CAD build for the part. Positions are in the model's coordinates, mm. Give positions to 0.01 mm unless a question says otherwise; leave off trailing zeros. Write each loop counter-clockwise with the first axis right and the second up, starting at its lowest first coordinate (ties: lowest second). Pieces come first, ordered by that corner, then holes. Notation, with made-up numbers: M -0.75,42 L 32.25,42 A26 cw 32.25,57 Z; hole C -15.75,14.5 d7. An arc over 180 degrees is marked long. One line per question, with ' | ' between items. Start each with the question number.
1. Wall check: L1, parallel to X at y = 0, z = -1.15; L2, parallel to Z at x = 19, y = 150. Give the ranges that are in metal, low to high.
2. Cut at A-A, the plane y = 53. Write the cut outline in (x, z) (3 decimals), then the cut area to 3 significant figures.
3. Flat gauge pins, fed straight in: pin 1 (1.2 mm diameter, centred on x = 18.5, y = 52.5, fed in from +Z); pin 2 (0.9 mm diameter, centred on x = 0, y = 0, fed in from +Z); pin 3 (3 mm diameter, centred on x = 0, y = 177.44, fed in from +Z). Where does each tip first touch, or does it go through?
```python
from build123d import *

# Parameters (mm, degrees)
F0_W     = 49.8404
F0_H     = 183.4444
F0_R     = 1.5
F0_R_2   = 1.375
F1_DEPTH = 0.5
F2_W     = 49.8404
F2_H     = 183.4444
F2_R     = 1.375
F3_DEPTH = 3
F4_W     = 2.381
F4_H     = 183.4444
F5_DEPTH = 0.4


with BuildPart() as f1:
    # F0 (on Top) → F1 (new body)
    with BuildSketch(Plane.XY):
        with Locations((21.9202, 88.7222)):
            Rectangle(F0_W, F0_H)
        Circle(F0_R, mode=Mode.SUBTRACT)
        with Locations((43.8404, 0)):
            Circle(F0_R_2, mode=Mode.SUBTRACT)
        with Locations((0, 177.4444)):
            Circle(F0_R_2, mode=Mode.SUBTRACT)
        with Locations((43.8404, 177.4444)):
            Circle(F0_R, mode=Mode.SUBTRACT)
    extrude(amount=F1_DEPTH)

    # F2 (on face) → F3 (join)
    with BuildSketch(Plane(origin=(0, 0, 0), x_dir=(1, 0, 0), z_dir=(0, 0, -1))):
        with Locations((21.9202, -88.7222)):
            Rectangle(F2_W, F2_H)
        with Locations((0, -177.4444)):
            Circle(F2_R, mode=Mode.SUBTRACT)
        with Locations((43.8404, 0)):
            Circle(F2_R, mode=Mode.SUBTRACT)
    extrude(amount=F3_DEPTH)

    # F4 (on face) → F5 (cut)
    with BuildSketch(Plane.XY.offset(0.5)):
        with Locations((5.8755, 88.7222)):
            Rectangle(F4_W, F4_H)
        with Locations((18.5415, 88.7222)):
            Rectangle(F4_W, F4_H)
        with Locations((22.6395, 88.7222)):
            Rectangle(F4_W, F4_H)
        with Locations((35.3055, 88.7222)):
            Rectangle(F4_W, F4_H)
    extrude(amount=-F5_DEPTH, mode=Mode.SUBTRACT)


solid = f1.part
```
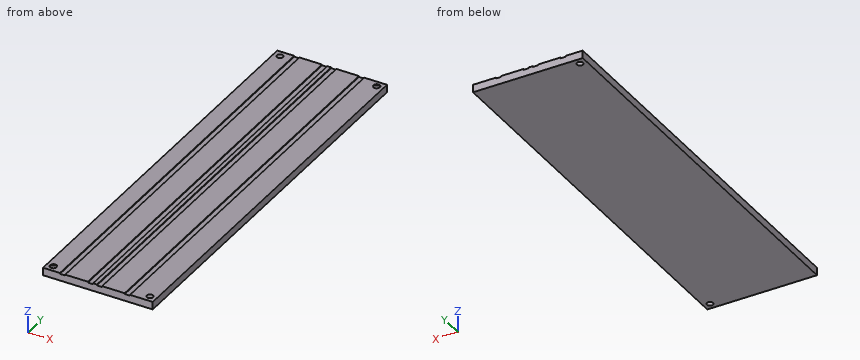
Here are the results:
1) L1: -3 to 42.47, 45.22 to 46.84 | L2: -3 to 0.1
2) outline: M -3,-3 L 46.84,-3 L 46.84,0.5 L 36.496,0.5 L 36.496,0.1 L 34.115,0.1 L 34.115,0.5 L 23.83,0.5 L 23.83,0.1 L 21.449,0.1 L 21.449,0.5 L 19.732,0.5 L 19.732,0.1 L 17.351,0.1 L 17.351,0.5 L 7.066,0.5 L 7.066,0.1 L 4.685,0.1 L 4.685,0.5 L -3,0.5 Z | area: 171 mm^2
3) pin 1: z = 0.1 | pin 2: z = 0 | pin 3: z = 0.5
